Input: dimensioned drawing with shaded views. Units: mm. Origin: part minimum x, y, z. Give positions to 0.01 mm unless a question says otherwise; leave off trailing zeros. Loops run counter-clockwise (first coordinate to the right, second up) from the corner with the lowest first, then second, coordinate; pieces in that order, holes last.
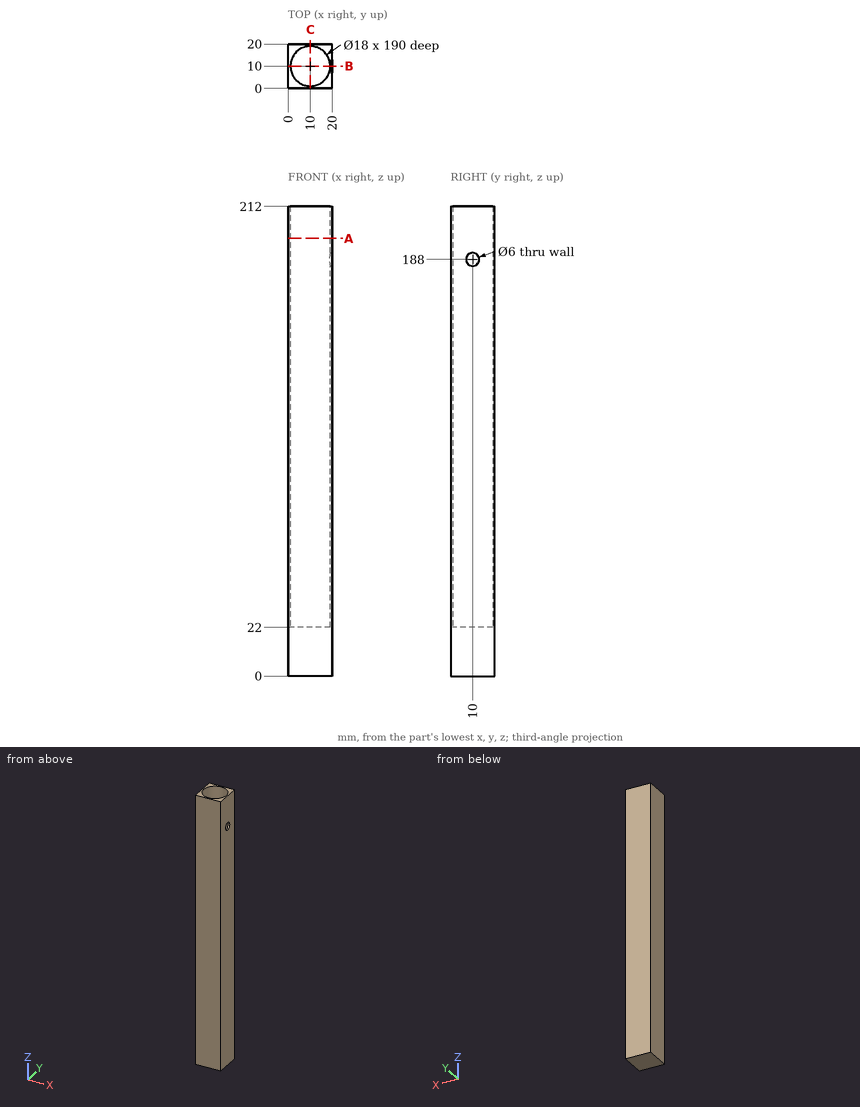
Item 1: Section query B-B on y = 10. Return loops of the section in (x, z).
Values follow:
outline: (0, 0) - (20, 0) - (20, 185) - (19, 185) - (19, 22) - (1, 22) - (1, 212) - (0, 212) - close; (19, 191) - (20, 191) - (20, 212) - (19, 212) - close
Item 2: Ray query, probe 1 along Y at (x, z) = (10, 117.5); probe 2 along Z at (x, y) = (19.2, 10); probe 3 along Y at (x, z) = (19.35, 188). Return the intervals inside material, ascending.
Values follow:
probe 1: y = 0 to 1, 19 to 20
probe 2: z = 0 to 185, 191 to 212
probe 3: y = 0 to 7, 13 to 20
Item 3: Section query C-C on x = 10. Return loops of the section in (y, z), plus the area to 3 significant figures.
Values follow:
outline: (0, 0) - (20, 0) - (20, 212) - (19, 212) - (19, 22) - (1, 22) - (1, 212) - (0, 212) - close
area: 820 mm2
Item 4: Section query A-A on z = 197.5. Return loops of the section in (x, y), plus the area to 3 significant figures.
Values follow:
outline: (0, 0) - (20, 0) - (20, 20) - (0, 20) - close; hole circle Ø18 at (10, 10)
area: 146 mm2
Item 5: Pin query (flat end, axial travel): pin 1 (1.5 mm diameter, centred on x = 11.5, y = 18, fed in from +Z). Return the tip coordinate at first contact, or that it passes through.
Values follow:
pin 1: stops at z = 22
